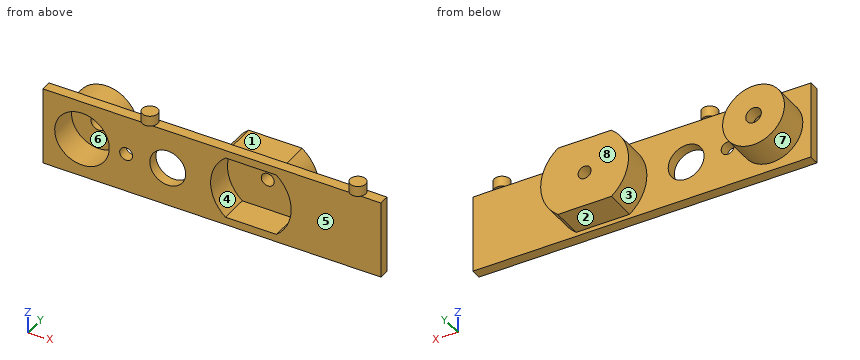
```python
from build123d import *

# Parameters (mm, degrees)
SKETCH_1_W               = 65
SKETCH_1_H               = 15
EXTRUDE_1_DEPTH          = 2
SKETCH_2_R               = 1.25
SKETCH_2_R_2             = 3.45
SKETCH_2_R_3             = 1.5
CUT_EXTRUDE_1_DEPTH      = 2
SKETCH_4_R               = 1.5
EXTRUDE_2_DEPTH          = 2
SKETCH_5_R               = 5.95
SKETCH_5_R_2             = 5.25
EXTRUDE_3_DEPTH          = 6
SKETCH_5_8_R             = 1.25
SKETCH_5_8_R_2           = 5.25
EXTRUDE_4_DEPTH          = 6
CUT_EXTRUDE_2_DEPTH      = 3.5
CUT_EXTRUDE_2_DEPTH_BACK = 42.548164821
SKETCH_5_11_R            = 1.25
SKETCH_5_11_R_2          = 5.25
SKETCH_2_3_R             = 1.5
CUT_EXTRUDE_3_DEPTH      = 8


with BuildPart() as part:
    # 草图1 → 凸台-拉伸1 (new body)
    with BuildSketch(Plane(origin=(0, 0, 0), x_dir=(1, 0, 0), z_dir=(0, 1, 0))):
        with Locations((-7.5, 0)):
            Rectangle(SKETCH_1_W, SKETCH_1_H)
    extrude(amount=EXTRUDE_1_DEPTH)

    # 草图2 → 切除-拉伸1 (cut)
    with BuildSketch(Plane(origin=(0, 0, 0), x_dir=(1, 0, 0), z_dir=(0, 1, 0))):
        with Locations(Location((0, 0, 0), (0, 0, 270))):
            Circle(SKETCH_2_R)
        with Locations(Location((-16, 0, 0), (0, 0, 90))):
            Circle(SKETCH_2_R_2)
        with Locations(Location((-24, 0, 0), (0, 0, 90))):
            Circle(SKETCH_2_R)
        with Locations(Location((-32.5, 0, 0), (0, 0, 270))):
            Circle(SKETCH_2_R_3)
    extrude(amount=CUT_EXTRUDE_1_DEPTH, mode=Mode.SUBTRACT)

    # 草图4 → 凸台-拉伸2 (add)
    with BuildSketch(Plane.XY.offset(7.5)):
        with Locations(Location((20, 1, 0), (0, 0, 221.810314896))):
            Circle(SKETCH_4_R)
        with Locations(Location((-20, 1, 0), (0, 0, 221.810314896))):
            Circle(SKETCH_4_R)
    extrude(amount=EXTRUDE_2_DEPTH)

    # 草图5 → 凸台-拉伸3 (add)
    # profile 1 of 2: a face of its own
    with BuildSketch(Plane(origin=(0, 2, 0), x_dir=(1, 0, 0), z_dir=(0, 1, 0))):
        with Locations(Location((-32.5, 0, 0), (0, 0, 270))):
            Circle(SKETCH_5_R)
        with Locations(Location((-32.5, 0, 0), (0, 0, 270))):
            Circle(SKETCH_5_R_2, mode=Mode.SUBTRACT)
    # profile 2 of 2: a face of its own
    with BuildSketch(Plane(origin=(0, 2, 0), x_dir=(1, 0, 0), z_dir=(0, 1, 0))):
        with BuildLine():
            Line((5.149029035, -6.7), (-5.149029035, -6.7))
            ThreePointArc((-5.149029035, -6.7), (-8.45, 0), (-5.149029035, 6.7))
            Line((-5.149029035, 6.7), (5.149029035, 6.7))
            ThreePointArc((5.149029035, 6.7), (8.45, 0), (5.149029035, -6.7))
        make_face()
        with BuildLine():
            Line((4.905354218, -6), (-4.905354218, -6))
            ThreePointArc((-4.905354218, -6), (-7.75, 0), (-4.905354218, 6))
            Line((-4.905354218, 6), (4.905354218, 6))
            ThreePointArc((4.905354218, 6), (7.75, 0), (4.905354218, -6))
        make_face(mode=Mode.SUBTRACT)
    extrude(amount=EXTRUDE_3_DEPTH)

    # 草图5<8> → 凸台-拉伸4 (add)
    # profile 1 of 2: a face of its own
    with BuildSketch(Plane(origin=(0, 2, 0), x_dir=(1, 0, 0), z_dir=(0, 1, 0))):
        with BuildLine():
            Line((4.905354218, -6), (-4.905354218, -6))
            ThreePointArc((-4.905354218, -6), (-7.75, 0), (-4.905354218, 6))
            Line((-4.905354218, 6), (4.905354218, 6))
            ThreePointArc((4.905354218, 6), (7.75, 0), (4.905354218, -6))
        make_face()
        with Locations(Location((0, 0, 0), (0, 0, 270))):
            Circle(SKETCH_5_8_R, mode=Mode.SUBTRACT)
    # profile 2 of 2: a face of its own
    with BuildSketch(Plane(origin=(0, 2, 0), x_dir=(1, 0, 0), z_dir=(0, 1, 0))):
        with Locations((-32.5, 0)):
            Circle(SKETCH_5_8_R_2)
    extrude(amount=EXTRUDE_4_DEPTH)

    # 草图5<11> → 切除-拉伸2 (cut, two sides: drawn at the far end of the back side and taken through both)
    # profile 1 of 2: a face of its own
    with BuildSketch(Plane(origin=(0, 2, 0), x_dir=(1, 0, 0), z_dir=(0, 1, 0)).offset(-CUT_EXTRUDE_2_DEPTH_BACK)):
        with BuildLine():
            Line((4.905354218, -6), (-4.905354218, -6))
            ThreePointArc((-4.905354218, -6), (-7.75, 0), (-4.905354218, 6))
            Line((-4.905354218, 6), (4.905354218, 6))
            ThreePointArc((4.905354218, 6), (7.75, 0), (4.905354218, -6))
        make_face()
        with Locations(Location((0, 0, 0), (0, 0, 270))):
            Circle(SKETCH_5_11_R, mode=Mode.SUBTRACT)
    # profile 2 of 2: a face of its own
    with BuildSketch(Plane(origin=(0, 2, 0), x_dir=(1, 0, 0), z_dir=(0, 1, 0)).offset(-CUT_EXTRUDE_2_DEPTH_BACK)):
        with Locations(Location((-32.5, 0, 0), (0, 0, 270))):
            Circle(SKETCH_5_11_R_2)
    extrude(amount=CUT_EXTRUDE_2_DEPTH + CUT_EXTRUDE_2_DEPTH_BACK, mode=Mode.SUBTRACT)

    # 草图2<3> → 切除-拉伸3 (cut)
    with BuildSketch(Plane(origin=(0, 0, 0), x_dir=(1, 0, 0), z_dir=(0, 1, 0))):
        with Locations(Location((-32.5, 0, 0), (0, 0, 270))):
            Circle(SKETCH_2_3_R)
    extrude(amount=CUT_EXTRUDE_3_DEPTH, mode=Mode.SUBTRACT)


solid = part.part
```
Here's how the part is built. I have some questions about the finished solid (model axes, mm). Face numbers are marked on the shaded views. A direction names the side the tool comes from. Coordinates: 2 decimals unless noted, no trailing zeros. Loops run counter-clockwise (first coordinate to the right, second up) from the corner with the lowest first, then second, coordinate; pieces in that order, holes last. Notation, with made-up numbers: (-9.5, -1) - (28.5, -1) arc R21 cw to (28.5, 38) - close; hole circle Ø1 at (-0.5, -0.5). An arc over 180 degrees is marked (long way). Return JSON: item names as keys, results as strings. Group by question number.
Item 1: If we section it at A-A on y = 6.5: Write out the boundary of the cut face in (x, z), and give its area (3 significant figures).
Item 2: If we section it at B-B on x = -16: Write out the boundary of the cut face in (y, z), and give its area (3 significant figures).
Item 3: Will these pins go through, and if not, where does the flat tip stop? P1, Ø3, axis at x = -24, z = 0, coming from the -Y side; P2, Ø2, axis at x = 1, z = -1.5, coming from the -Y side; P3, Ø0.6, axis at x = 5, y = 1, coming from the +Z side; P4, Ø4, axis at x = -16, z = 0, coming from the +Y side.
Item 4: If we section it at C-C on y = 1: Write out the boundary of the cut face in (x, z), and give its area (3 significant figures).
Item 5: We'd pull the mould along Z, two halves only. Please class the marked faces 6, 7 and 8: +Z half, -Z half, draft (parallel to the pull), parting line (faces both ways), or undercut.
Item 6: I need wall thicknesses on line 1 (Z direction, x = 4, y = 5); line 2 (Z direction, x = -24, y = 0.7); line 3 (Y direction, x = -17, z = 3.75). Which ranges of each line are inside material? Lowest first, please. Write a range as from..to.
Item 7: On a 3-axis mill with a long thin cutter (end or side, diameter ignored), from which of +Z, -Z, +X, -X, +Y, -Y can I reach the whole of each face in a straight line? I mean the marked faces 1, 2, 3, 4 and 5. Say none if no direction works.
Item 8: If we section it at D-D on z = 2.5: Write out the boundary of the cut face in (x, y), and give its area (3 significant figures).
Calculated:
{
 "1": {"outline": "circle Ø11.9 at (-32.5, 0); (-5.15, -6.7) - (5.15, -6.7) arc R8.45 ccw to (5.15, 6.7) - (-5.15, 6.7) arc R8.45 ccw to start; hole circle Ø3 at (-32.5, 0); hole circle Ø2.5 at (0, 0)", "area": "299 mm^2"},
 "2": {"outline": "(0, -7.5) - (2, -7.5) - (2, -3.45) - (0, -3.45) - close; (0, 3.45) - (2, 3.45) - (2, 7.5) - (0, 7.5) - close", "area": "16.2 mm^2"},
 "3": {"P1": "stops at y = 0", "P2": "stops at y = 5.5", "P3": "stops at z = 7.5", "P4": "passes through"},
 "4": {"outline": "(-40, -7.5) - (25, -7.5) - (25, 7.5) - (21.5, 7.5) - (21.5, 9.5) - (18.5, 9.5) - (18.5, 7.5) - (-18.5, 7.5) - (-18.5, 9.5) - (-21.5, 9.5) - (-21.5, 7.5) - (-40, 7.5) - close; hole circle Ø10.5 at (-32.5, 0); hole circle Ø2.5 at (-24, 0); hole circle Ø6.9 at (-16, 0); hole (-4.91, -6) - (4.91, -6) arc R7.75 ccw to (4.91, 6) - (-4.91, 6) arc R7.75 ccw to start", "area": "693 mm^2"},
 "5": {"face 6": "undercut", "face 7": "parting line", "face 8": "draft"},
 "6": {"line 1": "z = -6.7..-6, 6..6.7", "line 2": "z = -7.5..-1.25, 1.25..7.5", "line 3": "y = 0..2"},
 "7": {"face 1": "+Z, +X, -X, +Y", "face 2": "-Z, +X, -X, +Y", "face 3": "+Y", "face 4": "-Y", "face 5": "-Z, +X, -X, -Y"},
 "8": {"outline": "(-40, 0) - (-37.12, 0) - (-37.12, 5.5) - (-27.88, 5.5) - (-27.88, 0) - (-18.38, 0) - (-18.38, 2) - (-27.1, 2) - (-27.1, 8) - (-37.9, 8) - (-37.9, 2) - (-40, 2) - close; (-13.62, 0) - (-7.34, 0) - (-7.34, 5.5) - (7.34, 5.5) - (7.34, 0) - (25, 0) - (25, 2) - (8.07, 2) - (8.07, 8) - (-8.07, 8) - (-8.07, 2) - (-13.62, 2) - close", "area": "151 mm^2"}
}
